Verification items for the finished model (mm, model axes). A direction names the side the tool comes from. Give positions to 0.01 mm unless a question says otherwise; leave off trailing zeros. Order: outer loops, then holes, each group sorted by start corner. A loop starts at its lowest first (then second) coordinate and runs counter-clockwise, first axis right, second up. Notation, with made-up numbers: (-10.5, -34) - (0.5, -34) arc R23 ccw to (0.5, -21) - close; hole circle Ø6 at (-31.75, -22). An arc over 180 degrees is marked (long way). Answer as a JSON object with one key per item and string values. Group by question number.
(1) Thickness scan on line 1 (Z direction, x = -17.25, y = -3.75); line 2 (Y direction, x = -15, z = 36.25); line 3 (X direction, y = 5.75, z = 7). Record the ranges inside material, lowest first.
(2) Section check B-B (z = 33). Count the separate pieces of the cut face and the enclosed holes in it, then the cut area to 3 significant figures.
(3) Section check A-A (x = 0). Record the boundary of the cut face in (y, z).
(4) Depth check by flat-ended pin: pin 1 Ø1 at (y, z) = (7, 12.5) entering from -X; pin 2 Ø1 at (y, z) = (-3.5, 22.5) entering from +X; pin 3 Ø1.5 at (y, z) = (-3, 10) entering from -X. Enter the tip coordinate at first touch or a pass-through.
(5) Section check C-C (y = 0.5). Record the boundary of the cut face in (x, z), then the cut area to 3 significant figures.
(6) Access from +Z, -Z, +X, -X, +Y, -Y to the whole of each face (thin tool, end or side, straight path). Record for faces 4 (the face through (-17.196, 4.289, 20.175)), 5 (the face through (-5, 10, 20)).
(7) Mould release check, pull along Y, two halves, no side actions. Record for faces 1 (the face through (-17.5, 0.1, 3.8)), 2 (the face through (5, 7, 20)), 3 (the face through (-21.99, 7.15, 20.28)): +Y half, -Y half, draft (parallel to the pull), parting line (faces both ways), or undercut.
Autodesk Inventor part; units mm, degrees
ref_plane "YZ Plane" through (0, 0, 0) normal (1, 0, 0) x (0, 1, 0)
ref_plane "XZ Plane" through (0, 0, 0) normal (0, 1, 0) x (-1, 0, 0)
ref_plane "XY Plane" through (0, 0, 0) normal (0, 0, 1) x (1, 0, 0)
sketch "Sketch1" plane through (0, 0, 0) normal (0, 0, 1) x (1, 0, 0)
  line L0 (-25, 10) -> (25, 10)
  line L1 (25, 10) -> (25, -10)
  line L2 (25, -10) -> (-25, -10)
  line L3 (-25, -10) -> (-25, 10)
  line L4 (-25, 10) -> (25, -10) construction
  line L5 (25, 10) -> (-25, -10) construction
  point P0 (0, 0)
  dimension "d0" = 50
  dimension "d1" = 20
extrude "Extrusion1" add sketch "Sketch1" along normal blind 40
sketch "Sketch2" plane through (0, 0, 40) normal (0, 0, 1) x (1, 0, 0)
  circle A0 centre (-15, 0) radius 2.5
  line L0 (-25, 10) -> (-25, -10)
  line L1 (-25, -10) -> (25, -10)
  point P0 (0, 0)
  dimension "d4" = 5
  dimension "d5" = 10
  dimension "d6" = 10
extrude "Extrusion2" cut sketch "Sketch2" against normal through all
sketch "Sketch3" plane through (25, -10, 0) normal (1, 0, 0) x (0, 0, -1)
  line L0 (-32.5, 4) -> (-7.5, 4)
  line L1 (-7.5, 4) -> (-7.5, 16)
  line L2 (-7.5, 16) -> (-32.5, 16)
  line L3 (-32.5, 16) -> (-32.5, 4)
  line L4 (-32.5, 4) -> (-7.5, 16) construction
  line L5 (-7.5, 4) -> (-32.5, 16) construction
  point P0 (0, 10)
  point P1 (-20, 10)
  dimension "d9" = 25
  dimension "d10" = 12
extrude "Extrusion3" cut sketch "Sketch3" against normal blind 44
full round fillet "Full Round Fillet1" first side at (10.3333, 6, 15.8333) centre faces at (-19, -2, 15.8333) second side at (10.3333, -6, 24.1667)
full round fillet "Full Round Fillet2" first side at (8.3333, 10, 13.3333) centre faces at (-25, 3.3333, 13.3333) second side at (-8.3333, -10, 13.3333)
sketch "Sketch4" plane through (25, -10, 0) normal (1, 0, 0) x (0, 0, -1)
  line L0 (-40, 0) -> (-40, 20)
  line L1 (0, 20) -> (0, 0)
  line L2 (-40, 20) -> (0, 20)
  line L3 (0, 20) -> (0, 0)
  line L4 (0, 0) -> (-40, 0)
  line L5 (-40, 0) -> (-40, 20)
  point P0 (0, 10)
extrude "Extrusion4" cut sketch "Sketch4" against normal blind 20
sketch "Sketch5" plane through (0, 0, 40) normal (0, 0, 1) x (1, 0, 0)
  line L0 (5, 10) -> (-15, 10)
  line L1 (5, -10) -> (5, 10)
  point P0 (0, 0)
  point P1 (0, 5)
  dimension "d15" = 5
  dimension "d16" = 5
hole "Hole1" at (0, 5, 40) direction (0, 0, -1) diameter 5 end through all
properties part number "3rd arm"
Solutions:
{
 "1": {"line 1": "z = 0 to 7.5, 32.5 to 40", "line 2": "y = -10 to -2.5, 2.5 to 10", "line 3": "x = -23.18 to -2.38, 2.38 to 5"},
 "2": {"separate pieces": "1", "enclosed holes": "2", "area": "518 mm2"},
 "3": {"outline": "(-10, 0) - (2.5, 0) - (2.5, 7.5) - (-6, 7.5) - (-6, 32.5) - (2.5, 32.5) - (2.5, 40) - (-10, 40) - close; (7.5, 0) - (10, 0) - (10, 40) - (7.5, 40) - close"},
 "4": {"pin 1": "stops at x = -22.6", "pin 2": "stops at x = -17.47", "pin 3": "stops at x = -24.74"},
 "5": {"outline": "(-24.99, 0) - (-17.45, 0) - (-17.45, 7.5) - (-18.98, 7.5) - (-18.98, 32.5) - (-17.45, 32.5) - (-17.45, 40) - (-24.99, 40) - close; (-12.55, 0) - (5, 0) - (5, 7.5) - (-12.55, 7.5) - close; (-12.55, 32.5) - (5, 32.5) - (5, 40) - (-12.55, 40) - close", "area": "527 mm2"},
 "6": {"face 4": "+X", "face 5": "+Z, -Z, +X, -X, +Y"},
 "7": {"face 1": "undercut", "face 2": "draft", "face 3": "+Y half"}
}
